Input: part model. Units: mm. Frame: model coordinates. Face numbers are marked on the shaded views. Coordinates: 2 decimals unless noted, no trailing zeros. Order: outer loops, then holes, each group sorted by start corner. A loop starts at its lowest first (then second) coordinate and runs counter-clockwise, first axis right, second up. Notation, with made-up numbers: (89, -8) -> (103, -8) arc R17 ccw to (103, 21) -> close; hole circle Ø8 at (-11, 7.25). An arc over 180 degrees is marked (long way). Write each question's results on one line, items separated by ' | '.
```python
from build123d import *
from build123d.topology import SkipClean

# Parameters (mm, degrees)
SKETCH2_R               = 21.8
BOSS_EXTRUDE1_DEPTH     = 41
BOSS_EXTRUDE2_DEPTH     = 41
CUT_EXTRUDE1_REACH      = 65.696
CUT_EXTRUDE1_END_RADIUS = 17.5
CUT_EXTRUDE2_START      = -2
CUT_EXTRUDE2_DEPTH      = 3.460986
SKETCH6_R               = 21.8
BOSS_EXTRUDE3_DEPTH     = 3


with BuildPart() as part:
    # Sketch2 → Boss-Extrude1 (new body)
    with BuildSketch(Plane(origin=(0, 0, 0), x_dir=(1, 0, 0), z_dir=(0, 1, 0))):
        with Locations(Location((0, 0, 0), (0, 0, 270))):
            Circle(SKETCH2_R)
        with BuildLine():
            Line((-1.626404494, -19.231349626), (-1.5, -17.736685147))
            ThreePointArc((-1.5, -17.736685147), (0, -17.8), (1.5, -17.736685147))
            Line((1.5, -17.736685147), (1.626404494, -19.231349626))
            ThreePointArc((1.626404494, -19.231349626), (12.767961734, -14.473049201), (18.878439522, -4.011797753))
            Line((18.878439522, -4.011797753), (17.41120329, -3.7))
            ThreePointArc((17.41120329, -3.7), (17.615608663, -2.555451317), (17.74485841, -1.4))
            Line((17.74485841, -1.4), (20.037733373, -1.580898876))
            ThreePointArc((20.037733373, -1.580898876), (20.1, 0), (20.037733373, 1.580898876))
            Line((20.037733373, 1.580898876), (17.74485841, 1.4))
            ThreePointArc((17.74485841, 1.4), (17.615608663, 2.555451317), (17.41120329, 3.7))
            Line((17.41120329, 3.7), (18.878439522, 4.011797753))
            ThreePointArc((18.878439522, 4.011797753), (0, 19.3), (-18.878439522, 4.011797753))
            Line((-18.878439522, 4.011797753), (-17.41120329, 3.7))
            ThreePointArc((-17.41120329, 3.7), (-17.615608663, 2.555451317), (-17.74485841, 1.4))
            Line((-17.74485841, 1.4), (-20.037733373, 1.580898876))
            ThreePointArc((-20.037733373, 1.580898876), (-20.1, 0), (-20.037733373, -1.580898876))
            Line((-20.037733373, -1.580898876), (-17.74485841, -1.4))
            ThreePointArc((-17.74485841, -1.4), (-17.615608663, -2.555451317), (-17.41120329, -3.7))
            Line((-17.41120329, -3.7), (-18.878439522, -4.011797753))
            ThreePointArc((-18.878439522, -4.011797753), (-12.767961734, -14.473049201), (-1.626404494, -19.231349626))
        make_face(mode=Mode.SUBTRACT)
    extrude(amount=BOSS_EXTRUDE1_DEPTH)

    # Sketch3 → Boss-Extrude2 (add)
    with SkipClean():  # the faces are left unmerged after this step: merging them gives an invalid solid
        with BuildSketch(Plane.XZ):
            with BuildLine():
                Line((11, -18.82126457), (11, -13.610657589))
                ThreePointArc((11, -13.610657589), (0, -17.5), (-11, -13.610657589))
                Line((-11, -13.610657589), (-11, -18.82126457))
                ThreePointArc((-11, -18.82126457), (0, -21.8), (11, -18.82126457))
            make_face()
        extrude(amount=-BOSS_EXTRUDE2_DEPTH)

    # Cut-Extrude1: up to this cylinder (the profile starts outside it)
    with SkipClean():  # the faces are left unmerged after this step: merging them gives an invalid solid
        cut_extrude1_end = Plane(origin=(0, 4.031925, 0), z_dir=(0, -1, 0)) * Cylinder(CUT_EXTRUDE1_END_RADIUS, 167.392, mode=Mode.PRIVATE)
        # Sketch4 → Cut-Extrude1 (cut, up to the surface)
        with BuildSketch(Plane(origin=(0, 0, -21.8), x_dir=(-1, 0, 0), z_dir=(0, 0, -1)), mode=Mode.PRIVATE) as cut_extrude1_sk1:
            with BuildLine():
                Line((-9.5, 0), (9.5, 0))
                ThreePointArc((9.5, 0), (0, 9.5), (-9.5, 0))
            make_face()
        cut_extrude1_tool1 = extrude(cut_extrude1_sk1.sketch, amount=-CUT_EXTRUDE1_REACH, mode=Mode.PRIVATE) - cut_extrude1_end
        add(cut_extrude1_tool1.solids().sort_by_distance((0, 4.031925, -21.8))[0], mode=Mode.SUBTRACT)

    # Sketch5 → Cut-Extrude2 (cut)
    with SkipClean():  # the faces are left unmerged after this step: merging them gives an invalid solid
        with BuildSketch(Plane.XY.offset(-17.5).offset(CUT_EXTRUDE2_START)):
            with BuildLine():
                ThreePointArc((-7, 20.3), (0, 13.3), (7, 20.3))
                Line((7, 20.3), (7, 29.3))
                Line((7, 29.3), (-7, 29.3))
                Line((-7, 29.3), (-7, 20.3))
            make_face()
        extrude(amount=CUT_EXTRUDE2_DEPTH, mode=Mode.SUBTRACT)

    # Sketch6 → Boss-Extrude3 (add)
    with SkipClean():  # the faces are left unmerged after this step: merging them gives an invalid solid
        with BuildSketch(Plane(origin=(0, 41, 0), x_dir=(1, 0, 0), z_dir=(0, 1, 0))):
            with Locations(Location((0, 0, 0), (0, 0, 64.165074802))):
                Circle(SKETCH6_R)
        extrude(amount=BOSS_EXTRUDE3_DEPTH)


solid = part.part
```
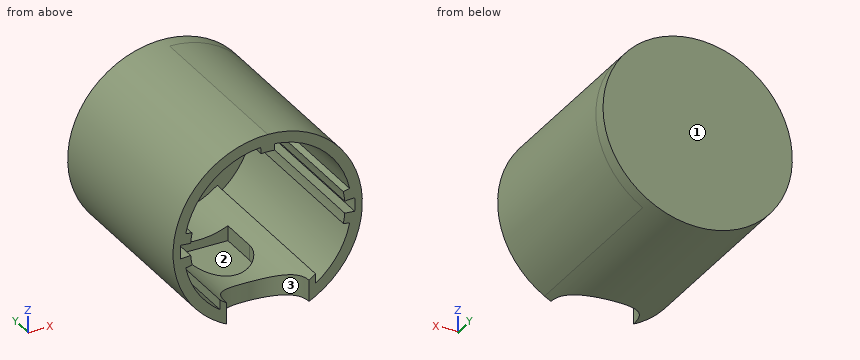
(1) Pin query (flat end, axial travel): P1, Ø1.8, axis at y = 13, z = -14, coming from the +X side (3 decimals); P2, Ø5, axis at x = -5, y = 4.5, coming from the -Z side; P3, Ø4, axis at x = 2, z = -17, coming from the -Y side. Return the tip coordinate at first contact, or that it passes through.
Return value:
P1: x = 17.425 | P2: z = 17.78 | P3: y = 8.62
(2) Line query: line 1 along Y through (x, z) = (-7.5, -2); line 2 along X through (y, z) = (33, -11); line 3 along X through (y, z) = (10.5, -13.5). Output: solid intervals per line, ascending. Write a range as from..to.
Return value:
line 1: 41..44 | line 2: -18.82..-15.86, 15.86..18.82 | line 3: -17.12..-13.79, 13.79..17.12
(3) Cut plane B-B, the plane z = 0. Return loops of the section in (x, y).
Return value:
outline: (-21.8, 0) -> (-20.1, 0) -> (-20.1, 41) -> (20.1, 41) -> (20.1, 0) -> (21.8, 0) -> (21.8, 44) -> (-21.8, 44) -> close
(4) Mould query, pull axis X, two halves, no side actions, for the marked faces 1, 2 and 3. Classes: +X half, -X half, draft (parallel to the pull), parting line (faces both ways), or undercut.
Return value:
face 1: draft | face 2: undercut | face 3: undercut
(5) Cut plane D-D, the plane x = 14. Return loops of the section in (y, z), plus the area to 3 significant figures.
Return value:
outline: (0, -16.71) -> (44, -16.71) -> (44, 16.71) -> (0, 16.71) -> (0, 13.28) -> (41, 13.28) -> (41, -13.28) -> (0, -13.28) -> close | area: 381 mm2
(6) Cut plane C-C, the plane y = 35.5. Return loops of the section in (x, z).
Return value:
outline: circle Ø43.6 at (0, 0); hole (-20.04, -1.58) -> (-17.74, -1.4) arc R17.8 ccw to (-17.41, -3.7) -> (-18.88, -4.01) arc R19.3 ccw to (-11, -15.86) -> (-11, -13.61) arc R17.5 ccw to (11, -13.61) -> (11, -15.86) arc R19.3 ccw to (18.88, -4.01) -> (17.41, -3.7) arc R17.8 ccw to (17.74, -1.4) -> (20.04, -1.58) arc R20.1 ccw to (20.04, 1.58) -> (17.74, 1.4) arc R17.8 ccw to (17.41, 3.7) -> (18.88, 4.01) arc R19.3 ccw to (1.63, 19.23) -> (1.5, 17.74) arc R17.8 ccw to (-1.5, 17.74) -> (-1.63, 19.23) arc R19.3 ccw to (-18.88, 4.01) -> (-17.41, 3.7) arc R17.8 ccw to (-17.74, 1.4) -> (-20.04, 1.58) arc R20.1 ccw to start
